Check sheet for the modelled part. Datum: model origin and axes. Units: mm. A direction names the side the tool comes from. Give positions to 0.01 mm unless a question says otherwise; leave off trailing zeros. Loops run counter-clockwise (first coordinate to the right, second up) from the corner with the lowest first, then second, coordinate; pieces in that order, holes last. Notation, with made-up numbers: (63, 37.5) -> (106, 37.5) arc R5 cw to (106, 42.5) -> close; hole circle Ø1 at (38.5, 76.5). An arc over 180 degrees is marked (long way). Answer as CSV lines item,"result". Start each with the question number.
(1) Section check C-C on z = 22.25. Enter the section's corners in (x, y) (3 decimals).
(2) Section check D-D on y = 11.5. Enter the section's corners in (x, z).
(3) Access from +Z, -Z, +X, -X, +Y, -Y to the whole of each face (thin tool, end or side, straight path). Record for faces 1 (the face through (0, 19.05, 13)), 2 (the face through (5.474, 6.306, 12.878)), 3 (the face through (0, 0, 13)).
(4) Gauge pin test, flat ends, axial feed: pin 1 Ø6 at (y, z) = (28.575, 12.7) entering from +X; pin 2 Ø5.5 at (y, z) = (32.5, 15.5) entering from -X; pin 3 Ø3.5 at (x, z) = (1.5, 8.5) entering from +Y. Record the tip position at first contact, or that the pin passes through.
(5) Release check for a two-part mould opening along X. For faces 4 (the face through (-12.7, 19, 13)), 5 (the face through (0, 15.875, 13)), 6 (the face through (5.5, 12.7, 12.9)), 7 (the face through (-9.481, 33.574, 13.356)) record: pulls with the +X half, pulls with the -X half, needs draft (parallel to the pull), parting line crosses it, or undercut.
(6) Section check B-B on x = 1.75. Enter the section's corners in (y, z) (3 decimals).
(7) Section check A-A on z = 12.7. Enter the section's corners in (x, y) (3 decimals).
(8) Material ranges on line 1 (Y direction, x = -10.5, z = 12.7); line 2 (X direction, y = 20.5, z = 8); line 3 (Y direction, x = -0.5, z = 17) (3 decimals), recorded low to high. Write a range as from..to.
from build123d import *

# Parameters (mm, degrees)
BOSS_EXTRUDE1_DEPTH     = 25.4
CUT_EXTRUDE1_DEPTH      = 48.519048812
F_3_8_CLEARANCE_HOLE1_D = 10.0838


with BuildPart() as part:
    # Sketch1 → Boss-Extrude1 (new body)
    with BuildSketch(Plane.XY):
        Polygon((-12.7, 0), (12.7, 0), (12.7, 38.1), (6.35, 38.1), (6.35, 19.05), (-6.35, 19.05), (-6.35, 38.1), (-12.7, 38.1), align=None)
    extrude(amount=BOSS_EXTRUDE1_DEPTH)

    # Sketch2 → Cut-Extrude1 (cut, through all)
    with BuildSketch(Plane.XY.offset(25.4)):
        Polygon((3.666174209, 15.875), (-3.666174209, 15.875), (-7.332348419, 9.525), (-3.666174209, 3.175), (3.666174209, 3.175), (7.332348419, 9.525), align=None)
    extrude(amount=-CUT_EXTRUDE1_DEPTH, mode=Mode.SUBTRACT)

    # 3/8 Clearance Hole1 (through all)
    with Locations(Plane.ZY.offset(12.7)):
        with Locations((12.7, 28.575)):
            Hole(F_3_8_CLEARANCE_HOLE1_D / 2)


solid = part.part
Working result:
1,outline,"(-12.7, 0) -> (12.7, 0) -> (12.7, 38.1) -> (6.35, 38.1) -> (6.35, 19.05) -> (-6.35, 19.05) -> (-6.35, 38.1) -> (-12.7, 38.1) -> close; hole (-7.332, 9.525) -> (-3.666, 3.175) -> (3.666, 3.175) -> (7.332, 9.525) -> (3.666, 15.875) -> (-3.666, 15.875) -> close"
2,outline,"(-12.7, 0) -> (-6.19, 0) -> (-6.19, 25.4) -> (-12.7, 25.4) -> close; (6.19, 0) -> (12.7, 0) -> (12.7, 25.4) -> (6.19, 25.4) -> close"
3,face 1,"+Z, -Z, +Y"
3,face 2,"+Z, -Z"
3,face 3,"+Z, -Z, +X, -X, -Y"
4,pin 1,"passes through"
4,pin 2,"stops at x = -12.7"
4,pin 3,"stops at y = 19.05"
5,face 4,"pulls with the -X half"
5,face 5,"undercut"
5,face 6,"undercut"
5,face 7,"needs draft"
6,outline,"(0, 0) -> (3.175, 0) -> (3.175, 25.4) -> (0, 25.4) -> close; (15.875, 0) -> (19.05, 0) -> (19.05, 25.4) -> (15.875, 25.4) -> close"
7,outline,"(-12.7, 0) -> (12.7, 0) -> (12.7, 23.533) -> (6.35, 23.533) -> (6.35, 19.05) -> (-6.35, 19.05) -> (-6.35, 23.533) -> (-12.7, 23.533) -> close; (-12.7, 33.617) -> (-6.35, 33.617) -> (-6.35, 38.1) -> (-12.7, 38.1) -> close; (6.35, 33.617) -> (12.7, 33.617) -> (12.7, 38.1) -> (6.35, 38.1) -> close; hole (-7.332, 9.525) -> (-3.666, 3.175) -> (3.666, 3.175) -> (7.332, 9.525) -> (3.666, 15.875) -> (-3.666, 15.875) -> close"
8,line 1,"y = 0..23.53, 33.62..38.1"
8,line 2,"x = -12.7..-6.35, 6.35..12.7"
8,line 3,"y = 0..3.175, 15.875..19.05"
